Design review of the part built by this model. Coordinates are the model's own, in mm. Coordinates: 2 decimals unless noted, no trailing zeros.
Q1. The part is to be moulded in two halves that separate along X. For faces 1 (the face through (82.134, 22.516, 172.55)), 2 (the face through (0, 20, 173)), say which applies: +X half, -X half, draft (parallel to the pull), parting line (faces both ways), or undercut.
Q2. To check wall thickness, follow probe 1 along Z at (x, y) = (90, 2.1); probe 2 along X at (y, z) = (3.5, 85); probe 3 along Z at (x, y) = (112, 1.55). State the ranges of each line that lie inside material, in increasing order.
Q3. Add section A-A, the plane y = 19. Give the number of separate pieces and of enclosed holes in the cut face, plus the area to 3 significant figures.
Q4. Clearance check with flat-ended pins moving along their axes: pin 1 Ø3.5 at (x, z) = (96, 295) entering from -Y; pin 2 Ø2 at (x, z) = (37.5, 208) entering from +Y. State where each tip first meets the part, or that it passes through.
from build123d import *

# Parameters (mm, degrees)
EXTRUDE_1_DEPTH       = 350
EXTRUDE_3_DEPTH       = 350
PATTERN_CURVE_1_DEPTH = 350
SKETCH_3_R            = 2.25
CUT_EXTRUDE_1_DEPTH   = 6
SKETCH_4_R            = 1.6
SKETCH_4_R_2          = 2.25
SKETCH_4_R_3          = 2.1
SKETCH_4_R_4          = 1.1
CUT_EXTRUDE_2_DEPTH   = 6


# Read off the part's stored shape, not the designer's step: the pattern curve step
with BuildPart() as part:
    # Sketch 1 → Extrude 1 (new body)
    with BuildSketch(Plane.XY):
        with BuildLine():
            Line((0, 40), (1.528979332, 40))
            ThreePointArc((1.528979332, 40), (2.225614441, 39.717425624), (2.528547087, 39.029399052))
            Line((2.528547087, 39.029399052), (3.5, 6))
            Line((3.5, 6), (118.5, 6))
            Line((118.5, 6), (119.471452913, 39.029399052))
            ThreePointArc((119.471452913, 39.029399052), (119.774385559, 39.717425624), (120.471020668, 40))
            Line((120.471020668, 40), (122, 40))
            Line((122, 40), (122, 0))
            Line((122, 0), (0, 0))
            Line((0, 0), (0, 40))
        make_face()
    extrude(amount=EXTRUDE_1_DEPTH)

    # Sketch 2 → Extrude 3 (add)
    with BuildSketch(Plane.XY.offset(350)):
        with BuildLine():
            Line((10.5, 39.5), (9.25, 6))
            Line((9.25, 6), (12.75, 6))
            Line((12.75, 6), (11.5, 39.5))
            ThreePointArc((11.5, 39.5), (11, 40), (10.5, 39.5))
        make_face()
    extrude(amount=-EXTRUDE_3_DEPTH)

    # Pattern Curve 1 outline → Pattern Curve 1 (add)
    with BuildSketch(Plane.XY):
        with BuildLine():
            ThreePointArc((21.5, 39.5), (21, 40), (20.5, 39.5))
            Line((20.5, 39.5), (19.25, 6))
            Line((19.25, 6), (22.75, 6))
            Line((22.75, 6), (21.5, 39.5))
        make_face()
        with BuildLine():
            Line((110.5, 39.5), (109.25, 6))
            Line((109.25, 6), (112.75, 6))
            Line((112.75, 6), (111.5, 39.5))
            ThreePointArc((111.5, 39.5), (111, 40), (110.5, 39.5))
        make_face()
        with BuildLine():
            Line((100.5, 39.5), (99.25, 6))
            Line((99.25, 6), (102.75, 6))
            Line((102.75, 6), (101.5, 39.5))
            ThreePointArc((101.5, 39.5), (101, 40), (100.5, 39.5))
        make_face()
        with BuildLine():
            Line((90.5, 39.5), (89.25, 6))
            Line((89.25, 6), (92.75, 6))
            Line((92.75, 6), (91.5, 39.5))
            ThreePointArc((91.5, 39.5), (91, 40), (90.5, 39.5))
        make_face()
        with BuildLine():
            Line((80.5, 39.5), (79.25, 6))
            Line((79.25, 6), (82.75, 6))
            Line((82.75, 6), (81.5, 39.5))
            ThreePointArc((81.5, 39.5), (81, 40), (80.5, 39.5))
        make_face()
        with BuildLine():
            Line((70.5, 39.5), (69.25, 6))
            Line((69.25, 6), (72.75, 6))
            Line((72.75, 6), (71.5, 39.5))
            ThreePointArc((71.5, 39.5), (71, 40), (70.5, 39.5))
        make_face()
        with BuildLine():
            Line((60.5, 39.5), (59.25, 6))
            Line((59.25, 6), (62.75, 6))
            Line((62.75, 6), (61.5, 39.5))
            ThreePointArc((61.5, 39.5), (61, 40), (60.5, 39.5))
        make_face()
        with BuildLine():
            Line((50.5, 39.5), (49.25, 6))
            Line((49.25, 6), (52.75, 6))
            Line((52.75, 6), (51.5, 39.5))
            ThreePointArc((51.5, 39.5), (51, 40), (50.5, 39.5))
        make_face()
        with BuildLine():
            Line((40.5, 39.5), (39.25, 6))
            Line((39.25, 6), (42.75, 6))
            Line((42.75, 6), (41.5, 39.5))
            ThreePointArc((41.5, 39.5), (41, 40), (40.5, 39.5))
        make_face()
        with BuildLine():
            Line((30.5, 39.5), (29.25, 6))
            Line((29.25, 6), (32.75, 6))
            Line((32.75, 6), (31.5, 39.5))
            ThreePointArc((31.5, 39.5), (31, 40), (30.5, 39.5))
        make_face()
    extrude(amount=PATTERN_CURVE_1_DEPTH)

    # Sketch 3 → Cut-Extrude 1 (cut)
    with BuildSketch(Plane.XZ):
        with Locations((26, 342)):
            Circle(SKETCH_3_R)
        with Locations((96, 342)):
            Circle(SKETCH_3_R)
        with Locations(Location((96, 8, 0), (0, 0, 180))):
            Circle(SKETCH_3_R)
        with Locations(Location((26, 8, 0), (0, 0, 180))):
            Circle(SKETCH_3_R)
    extrude(amount=-CUT_EXTRUDE_1_DEPTH, mode=Mode.SUBTRACT)

    # Sketch 4 → Cut-Extrude 2 (cut)
    with BuildSketch(Plane.XZ):
        with Locations((55, 25)):
            Circle(SKETCH_4_R)
        with Locations((90, 25)):
            Circle(SKETCH_4_R)
        with Locations((55, 85)):
            Circle(SKETCH_4_R)
        with Locations((90, 85)):
            Circle(SKETCH_4_R)
        with Locations((112, 25)):
            Circle(SKETCH_4_R_2)
        with Locations((55, 115)):
            Circle(SKETCH_4_R_3)
        with Locations((84.5, 115)):
            Circle(SKETCH_4_R)
        with Locations((112, 107)):
            Circle(SKETCH_4_R_2)
        with Locations((96, 320)):
            Circle(SKETCH_4_R_2)
        with Locations((96, 295)):
            Circle(SKETCH_4_R_2)
        with Locations((55, 140)):
            Circle(SKETCH_4_R_4)
        with Locations((55, 166)):
            Circle(SKETCH_4_R_4)
        with Locations((55, 195)):
            Circle(SKETCH_4_R)
        with Locations((84.5, 255)):
            Circle(SKETCH_4_R)
    extrude(amount=-CUT_EXTRUDE_2_DEPTH, mode=Mode.SUBTRACT)


solid = part.part
Here are the results:
1. face 1: undercut
1. face 2: -X half
2. probe 1: z = 0 to 23.4, 26.6 to 83.4, 86.6 to 350
2. probe 2: x = 0 to 53.4, 56.6 to 88.4, 91.6 to 122
2. probe 3: z = 0 to 22.75, 27.25 to 104.75, 109.25 to 350
3. separate pieces: 13
3. enclosed holes: 0
3. area: 11,900 mm2
4. pin 1: passes through
4. pin 2: stops at y = 6
